Part print with two shaded views. Sizes in mm from the minimum x, y, z corner. A direction names the side the tool comes from. Coordinates: 2 decimals unless noted, no trailing zeros. Loops run counter-clockwise (first coordinate to the right, second up) from the corner with the lowest first, then second, coordinate; pieces in that order, holes last. Notation, with made-up numbers: (40.5, 12.5) -> (56.5, 12.5) arc R21 ccw to (56.5, 25.5) -> close; hole circle Ø1 at (-8.75, -12.5). An arc over 180 degrees is marked (long way). Use one line per item in the form item = value.
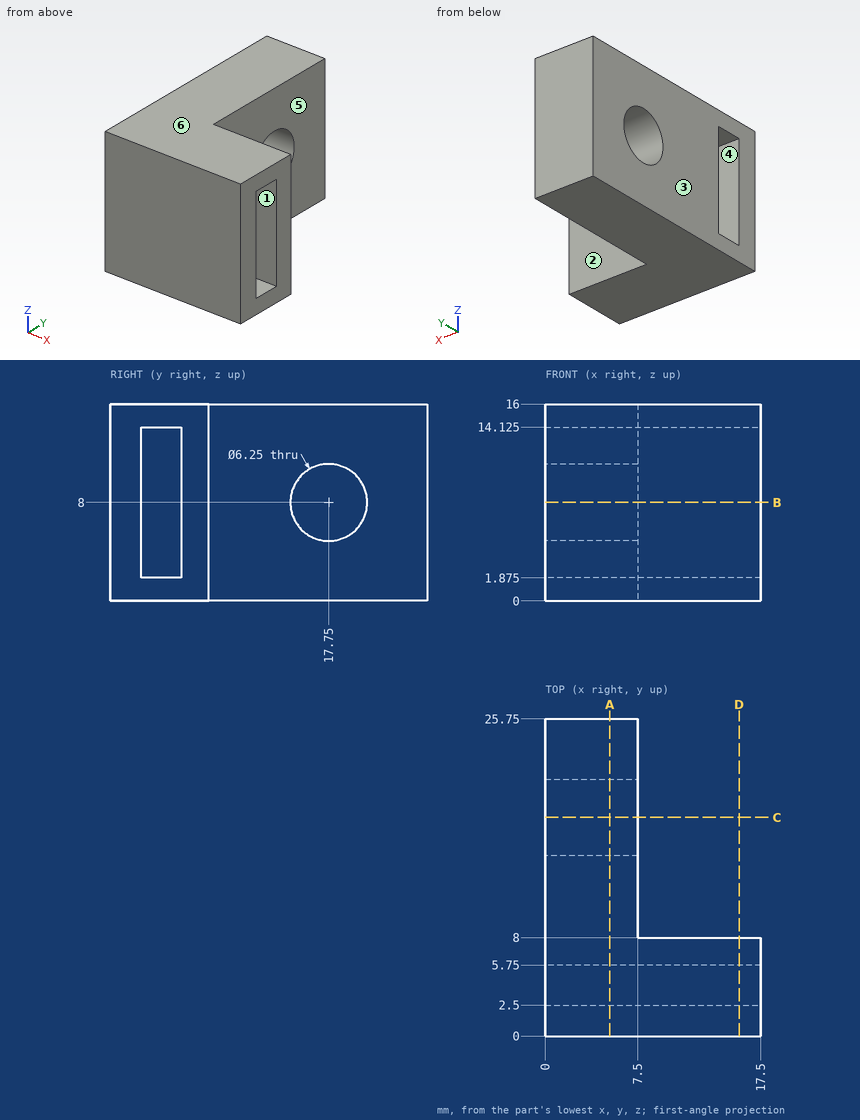
Q1. Band-saw the part on B-B, the plane z = 8. Write the cut outline in (x, y) (3 decimals), and give its area (3 significant figures).
Result:
outline = (0, 0) -> (17.5, 0) -> (17.5, 2.5) -> (0, 2.5) -> close; (0, 5.75) -> (17.5, 5.75) -> (17.5, 8) -> (7.5, 8) -> (7.5, 14.625) -> (0, 14.625) -> close; (0, 20.875) -> (7.5, 20.875) -> (7.5, 25.75) -> (0, 25.75) -> close
area = 169 mm2
Q2. Wall check: line 1 along Z through (x, y) = (4.5, 17.75) (3 decimals); line 2 along Y through (x, z) = (2.5, 12); line 3 along Y through (x, z) = (10.25, 2.5). Give the ranges that are in metal, low to high.
Result:
line_1 = 0 to 4.875, 11.125 to 16
line_2 = 0 to 2.5, 5.75 to 25.75
line_3 = 0 to 2.5, 5.75 to 8
Q3. Band-saw the part on A-A, the plane x = 5.25. Write the cut outline in (y, z) (3 decimals), and give its area (3 significant figures).
Result:
outline = (0, 0) -> (25.75, 0) -> (25.75, 16) -> (0, 16) -> close; hole (2.5, 1.875) -> (5.75, 1.875) -> (5.75, 14.125) -> (2.5, 14.125) -> close; hole circle Ø6.25 at (17.75, 8)
area = 342 mm2
Q4. Pin check, flat tips, straight feed: pin 1 Ø8 at (y, z) = (12.5, 11.5) entering from +X; pin 2 Ø5 at (y, z) = (17.75, 8) entering from -X. Stop position of each tip, or through.
Result:
pin_1 = 7.5
pin_2 = through
Q5. Mould opens along Z. For the marked faces 4, 5 and 6 say: released by +Z, released by -Z, zero draft, split by the parting line, or undercut.
Result:
face_4 = undercut
face_5 = zero draft
face_6 = released by +Z
Q6. Which spindle directions (+Z, -Z, +X, -X, +Y, -Y) get a long thin tool onto all of the face, cutting with end or side? Do the marked faces 1, 2 and 3. Say none if no direction does.
Result:
face_1 = +X, -X
face_2 = +Z, -Z, +X, +Y
face_3 = +Z, -Z, -X, +Y, -Y
Q7. Band-saw the part on D-D, the plane x = 15.75. Write the cut outline in (y, z) (3 decimals), and give its area (3 significant figures).
Result:
outline = (0, 0) -> (8, 0) -> (8, 16) -> (0, 16) -> close; hole (2.5, 1.875) -> (5.75, 1.875) -> (5.75, 14.125) -> (2.5, 14.125) -> close
area = 88.2 mm2
Q8. Band-saw the part on C-C, the plane y = 17.75. Write the cut outline in (x, z) (3 decimals), and give its area (3 significant figures).
Result:
outline = (0, 0) -> (7.5, 0) -> (7.5, 4.875) -> (0, 4.875) -> close; (0, 11.125) -> (7.5, 11.125) -> (7.5, 16) -> (0, 16) -> close
area = 73.1 mm2
